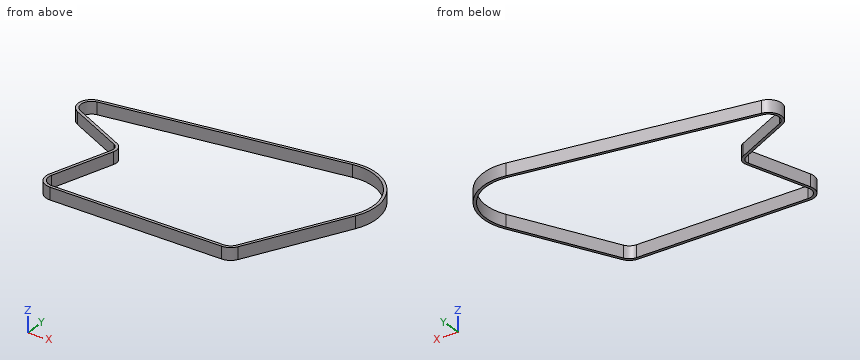
from build123d import *

# Parameters (mm, degrees)
EXTRUDE_THIN1_DEPTH      = 10
EXTRUDE_THIN1_DEPTH_BACK = 3


with BuildPart() as part:
    # Sketch2 → Extrude-Thin1 (new, two sides: drawn at the far end of the back side and taken through both)
    with BuildSketch(Plane.XY.offset(-EXTRUDE_THIN1_DEPTH_BACK)):
        with BuildLine():
            Line((242.697793623, 50.266129876), (-2.060433635, 13.847548997))
            ThreePointArc((-2.060433635, 13.847548997), (-13.833600307, 2.152092613), (-6.16977134, -12.56717636))
            Line((-6.16977134, -12.56717636), (51.739342618, -40.997269268))
            ThreePointArc((51.739342618, -40.997269268), (55.601208684, -45.108400995), (55.790656513, -50.745733973))
            Line((55.790656513, -50.745733973), (34.012493217, -115.021815701))
            ThreePointArc((34.012493217, -115.021815701), (35.902100375, -127.682924287), (47.298057776, -133.514428444))
            Line((47.298057776, -133.514428444), (228.230752902, -133.17848877))
            ThreePointArc((228.230752902, -133.17848877), (235.397453639, -131.189555479), (240.534146402, -125.810722655))
            Line((240.534146402, -125.810722655), (295.117855974, -24.338705573))
            ThreePointArc((295.117855974, -24.338705573), (291.932739821, 29.141852266), (242.697793623, 50.266129876))
        make_face()
        with BuildLine():
            Line((243.139315115, 47.298797948), (-1.618912142, 10.880217069))
            ThreePointArc((-1.618912142, 10.880217069), (-10.869257385, 1.69092991), (-4.847677482, -9.874209997))
            Line((-4.847677482, -9.874209997), (53.061436476, -38.304302905))
            ThreePointArc((53.061436476, -38.304302905), (58.371502316, -43.95710903), (58.631993081, -51.708441875))
            Line((58.631993081, -51.708441875), (36.853829786, -115.984523603))
            ThreePointArc((36.853829786, -115.984523603), (38.338521124, -125.932537492), (47.292487653, -130.514433615))
            Line((47.292487653, -130.514433615), (228.225182779, -130.178493941))
            ThreePointArc((228.225182779, -130.178493941), (233.85616193, -128.615760641), (237.892134815, -124.389534851))
            Line((237.892134815, -124.389534851), (292.475844387, -22.917517769))
            ThreePointArc((292.475844387, -22.917517769), (289.478088008, 27.417124903), (243.139315115, 47.298797948))
        make_face(mode=Mode.SUBTRACT)
    extrude(amount=EXTRUDE_THIN1_DEPTH + EXTRUDE_THIN1_DEPTH_BACK)


solid = part.part
Work out the finished part from the listing and answer in its coordinate system (mm). Coordinates: 2 decimals unless noted, no trailing zeros. Write each loop counter-clockwise with the first axis right and the second up, starting at its lowest first coordinate (ties: lowest second). Pieces come first, ordered by that corner, then holes. Notation, with made-up numbers: M 79.25,63.25 L 125.25,63.25 A16 ccw 125.25,80.25 Z; hole C 43,55 d6. An arc over 180 degrees is marked long. Use one line per item in the form item = value. Start each with the question number.
1. The part is cut by section A-A (z = 2.25). Give the vertices of the cut face in (x, y).
2. Straight lines are drawn through the part: probe 1 along Y at (x, z) = (13.5, -1.75); probe 2 along Y at (x, z) = (75.5, 5); probe 3 along X at (y, z) = (-94.5, 2.5). For each, find the intervals that lie inside material, in ascending order. Write a range as from..to.
3. The part is cut by section B-B (y = 38.5). Give the vertices of the cut face in (x, z), plus the area to 3 significant figures.
4. Each of these flat-tipped pins is pushed along its axis until it touches: P1, Ø1, axis at y = 8.5, z = 0.5, coming from the +X side; P2, Ø2, axis at y = -104.5, z = 1, coming from the -X side; P3, Ø5, axis at x = 85, z = -0.5, coming from the +Y side. Where does it stop, or does it pass through?
5. The part is cut by section C-C (x = 17.5). Give the vertices of the cut face in (y, z) (3 decimals).
Evaluation:
q1.outline = M -6.17,-12.57 L 51.74,-41 A8 cw 55.79,-50.75 L 34.01,-115.02 A14 ccw 47.3,-133.51 L 228.23,-133.18 A14 ccw 240.53,-125.81 L 295.12,-24.34 A51 ccw 242.7,50.27 L -2.06,13.85 A14 ccw Z; hole M -4.85,-9.87 L 53.06,-38.3 A11 cw 58.63,-51.71 L 36.85,-115.98 A11 ccw 47.29,-130.51 L 228.23,-130.18 A11 ccw 237.89,-124.39 L 292.48,-22.92 A48 ccw 243.14,47.3 L -1.62,10.88 A11 ccw Z
q2.probe_1 = -22.22..-18.88, 13.13..16.16
q2.probe_2 = -133.46..-130.46, 22.36..25.39
q2.probe_3 = 40.97..44.13, 253.97..257.38
q3.outline = M 163.62,-3 L 184.01,-3 L 184.01,10 L 163.62,10 Z; M 278.63,-3 L 283.44,-3 L 283.44,10 L 278.63,10 Z
q3.area = 328 mm^2
q4.P1 = 300.54
q4.P2 = 37.24
q4.P3 = 27.17
q5.outline = M -24.188,-3 L -20.846,-3 L -20.846,10 L -24.188,10 Z; M 13.725,-3 L 16.758,-3 L 16.758,10 L 13.725,10 Z
